Build history of the part. All positions in model axes, mm. A direction names the side the tool comes from. Give positions to 0.01 mm unless a question says otherwise; leave off trailing zeros. Write each loop counter-clockwise with the first axis right and the second up, starting at its lowest first coordinate (ties: lowest second). Pieces come first, ordered by that corner, then holes. Notation, with made-up numbers: (-34.5, 26.25) -> (0.5, 26.25) arc R25 cw to (0.5, 43.25) -> close; hole circle Ø7 at (29.5, 15.5). An arc over 180 degrees is marked (long way). Write item = value, one per line. Start each with the question number.
Q1. Saw through at D-D, the plane x = 6. List the corners of the cut face in (y, z), then the cut area to 3 significant figures.
Q2. Saw through at C-C, the plane x = -52. List the corners of the cut face in (y, z), then the cut area to 3 significant figures.
Q3. Wall check: line 1 (X direction, y = 1.5, z = -26.4); line 2 (Z direction, x = 27.4, y = 3.25); line 3 (X direction, y = 0, z = -26.4). Give the ranges that are in metal, low to high.
Q4. Drop flat-ended pins along their axis: P1, Ø10, axis at x = 5, z = -18, coming from the -Y side; P2, Ø3.5, axis at x = 27.4, z = -26.4, coming from the +Y side; P3, Ø1.8, axis at y = 1, z = -19, coming from the -X side; P4, Ø1.6, axis at y = -0.5, z = -17.5, coming from the +X side. Give the stop position or say it passes through.
Q5. Tool access for faces 4 (the face through (30.9, 0, -19)), 5 (the face through (-15, 4.5, -21)), 6 (the face through (29.9, -0.49, -28.85)), 7 (the face through (-2, 0, -29.9)): list every direction of +Z, -Z, +X, -X, +Y, -Y with a clear straight run to the whole face (end or side of a thin tool).
Q6. Saw through at B-B, the plane y = 2.25. List the corners of the cut face in (x, z), then the cut area to 3 significant figures.
Q7. Mould opens along X. For faces 1 (the face through (25.012, 1.458, -24.122)), 2 (the face through (-16, 2, -31)), 3 (the face through (30.688, 2.122, -29.617)) say: pulls with the +X half, pulls with the -X half, needs draft (parallel to the pull), parting line crosses it, or undercut.
Q8. Saw through at A-A, the plane z = -19.5. List the corners of the cut face in (x, y), then the cut area to 3 significant figures.
from build123d import *

# Parameters (mm, degrees)
SKETCH005_R      = 1.3
EXTRUDE003_DEPTH = 20
EXTRUDE039_DEPTH = 4
EXTRUDE042_DEPTH = 0.8
EXTRUDE002_DEPTH = 6
EXTRUDE037_DEPTH = 2


with BuildPart() as sweep001:
    # Sweep001: sweep along a path in Sketch034
    with BuildLine(Plane.XZ.offset(10)) as sweep001_path:
        Line((32, 11.999174), (32, 26.4))
        ThreePointArc((32, 26.4), (30.652691, 29.652691), (27.4, 31))
        Line((27.4, 31), (-60.9, 31))
    # Sketch035 → Sweep001 (sweep)
    with BuildSketch(Plane.YZ):
        Polygon((5.3, 29.4), (3.7, 31), (3.7, 32), (6, 32), (6, 29.4), align=None)
    sweep(path=sweep001_path.line)


with BuildPart() as fusion030:
    # Sketch005 → Extrude003 (new body)
    with BuildSketch(Plane.XZ.offset(5)):
        with Locations((27.4, 26.4)):
            Circle(SKETCH005_R)
    extrude(amount=-EXTRUDE003_DEPTH)


with BuildPart() as fusion030_1:
    # Extrude003 placement: moved
    add(fusion030.part.moved(Location((0, -4, 0))))

    # Fusion030: union Sweep001
    add(sweep001.part)


with BuildPart() as top003:
    # Sketch028 → Extrude039 (new body)
    with BuildSketch(Plane.XZ.offset(10)):
        with BuildLine():
            ThreePointArc((32, 26.4), (30.652691, 29.652691), (27.4, 31))
            Line((27.4, 31), (-60.9, 31))
            Line((-60.9, 31), (-60.9, 29))
            Line((-60.9, 29), (27.4, 29))
            ThreePointArc((30, 26.4), (29.238478, 28.238478), (27.4, 29))
            Line((30, 12), (30, 26.4))
            Line((32, 12), (30, 12))
            Line((32, 26.4), (32, 12))
        make_face()
    extrude(amount=EXTRUDE039_DEPTH)


with BuildPart() as top003_1:
    # Extrude039 placement: moved
    add(top003.part.moved(Location((0, 14.5, 0))))


with BuildPart() as top002:
    # Sketch031 → Extrude042 (new body)
    with BuildSketch(Plane.XZ.offset(10)):
        with BuildLine():
            ThreePointArc((32, 26.399981), (30.652691, 29.652672), (27.4, 30.999981))
            Line((27.4, 30.999981), (-60.9, 30.999981))
            Line((-60.9, 30.999981), (-60.9, 11.999981))
            Line((-60.9, 11.999981), (32, 11.999981))
            Line((32, 26.399981), (32, 11.999981))
        make_face()
    extrude(amount=EXTRUDE042_DEPTH)


with BuildPart() as top002_1:
    # Extrude042 placement: moved
    add(top002.part.moved(Location((0, 15.3, 0))))


with BuildPart() as screw_hole_top:
    # Sketch004 → Extrude002 (new body)
    with BuildSketch(Plane.XZ.offset(10)):
        with BuildLine():
            ThreePointArc((25.36776, 29), (25.066548, 24.066548), (30, 24.36776))
            Line((30, 24.36776), (30, 26.4))
            ThreePointArc((30, 26.4), (29.238478, 28.238478), (27.4, 29))
            Line((25.36776, 29), (27.4, 29))
        make_face()
    extrude(amount=-EXTRUDE002_DEPTH)


with BuildPart() as screw_hole_top_1:
    # Extrude002 placement: moved
    add(screw_hole_top.part.moved(Location((0, 8.5, 0))))


with BuildPart() as top:
    # Sketch029 → Extrude037 (new body)
    with BuildSketch(Plane.XZ.offset(10)):
        with BuildLine():
            ThreePointArc((30.9, 26.4), (29.874874, 28.874874), (27.4, 29.9))
            Line((27.4, 29.9), (-33, 29.9))
            Line((-33, 29.9), (-33, 29))
            Line((-33, 29), (27.4, 29))
            ThreePointArc((30, 26.4), (29.238478, 28.238478), (27.4, 29))
            Line((30, 12), (30, 26.4))
            Line((30.9, 12), (30, 12))
            Line((30.9, 26.4), (30.9, 12))
        make_face()
    extrude(amount=EXTRUDE037_DEPTH)


with BuildPart() as top_1:
    # Extrude037 placement: moved
    add(top.part.moved(Location((0, 10.5, 0))))

    # Fusion028: union top003, top002, screw hole top
    add(top003_1.part)
    add(top002_1.part)
    add(screw_hole_top_1.part)

    # Cut024: cut Fusion030
    add(fusion030_1.part, mode=Mode.SUBTRACT)


with BuildPart() as part_mirroring001:
    # Part__Mirroring001: instance of top
    add(top_1.part.mirror(Plane(origin=(0, 0, 0), x_dir=(0, 1, 0), z_dir=(0, 0, 1))))


solid = part_mirroring001.part
Report:
q1.outline = (-1.5, -29.9) -> (0.5, -29.9) -> (0.5, -31) -> (3.7, -31) -> (5.3, -29.4) -> (5.3, -12) -> (4.5, -12) -> (4.5, -29) -> (-1.5, -29) -> close
q1.area = 23.7 mm2
q2.outline = (0.5, -31) -> (3.7, -31) -> (5.3, -29.4) -> (5.3, -12) -> (4.5, -12) -> (4.5, -29) -> (0.5, -29) -> close
q2.area = 21.9 mm2
q3.line_1 = 24.1 to 26.1, 28.7 to 32
q3.line_2 = -31 to -27.7, -25.1 to -23.1
q3.line_3 = 24.1 to 26.1, 28.7 to 30.9
q4.P1 = 4.5
q4.P2 = 5.3
q4.P3 = 30
q4.P4 = 30.9
q5.face_4 = +Z, -Z, +X, -Y
q5.face_5 = +Z, -X, -Y
q5.face_6 = -Z, +X, -Y
q5.face_7 = -Z, +X, -X, -Y
q6.outline = (-60.9, -31) -> (27.4, -31) arc R4.6 ccw to (32, -26.4) -> (32, -12) -> (30, -12) -> (30, -24.37) arc R3.3 ccw (long way) to (25.37, -29) -> (-60.9, -29) -> close; hole circle Ø2.6 at (27.4, -26.4)
q6.area = 240 mm2
q7.face_1 = undercut
q7.face_2 = needs draft
q7.face_3 = pulls with the +X half
q8.outline = (-60.9, 4.5) -> (30, 4.5) -> (30, -1.5) -> (30.9, -1.5) -> (30.9, 0.5) -> (32, 0.5) -> (32, 3.7) -> (30.4, 5.3) -> (-60.9, 5.3) -> close
q8.area = 82.8 mm2
